Geometry check sheet. Reference: drawing and pictorial views, mm from the part's lowest x, y, z. Coordinates: 2 decimals unless noted, no trailing zeros. Loops run counter-clockwise (first coordinate to the right, second up) from the corner with the lowest first, then second, coordinate; pieces in that order, holes last. Notation, with made-up numbers: M -30,66 L 0,66 A22 ccw 0,102 Z; hole C 45.25,27.25 d3. An arc over 180 degrees is marked long. Write each question's results on one line, items separated by ' | '. Start each with the question number.
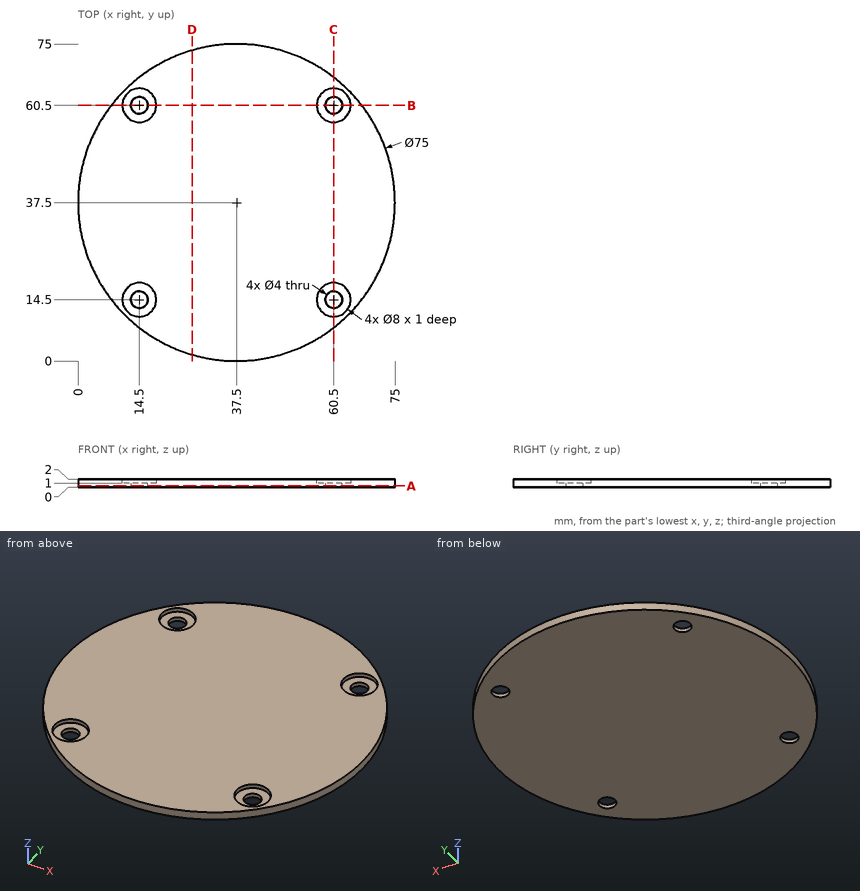
1) Thickness scan on probe 1 along Y at (x, z) = (14.5, 0.7); probe 2 along Y at (x, z) = (57, 1.5). Record the ranges inside material, lowest first.
2) Gauge pin test, flat ends, axial feed: P1, Ø2.5, axis at x = 14.5, y = 60.5, coming from the -Z side; P2, Ø6.5, axis at x = 60.5, y = 60.5, coming from the +Z side. Record the tip position at first contact, or that the pin passes through.
3) Section check B-B (y = 60.5). Enter the section's corners in (x, z).
4) Section check A-A (z = 0.35). Enter the section's corners in (x, y), then the cut area to 3 significant figures.
5) Section check D-D (x = 27). Enter the section's corners in (y, z), then the cut area to 3 significant figures.
Return value:
1) probe 1: y = 7.88 to 12.5, 16.5 to 58.5, 62.5 to 67.12 | probe 2: y = 5.47 to 12.56, 16.44 to 58.56, 62.44 to 69.53
2) P1: passes through | P2: stops at z = 1
3) outline: M 7.88,0 L 12.5,0 L 12.5,1 L 10.5,1 L 10.5,2 L 7.88,2 Z; M 16.5,0 L 58.5,0 L 58.5,1 L 56.5,1 L 56.5,2 L 18.5,2 L 18.5,1 L 16.5,1 Z; M 62.5,0 L 67.12,0 L 67.12,2 L 64.5,2 L 64.5,1 L 62.5,1 Z
4) outline: C 37.5,37.5 d75; hole C 14.5,14.5 d4; hole C 14.5,60.5 d4; hole C 60.5,14.5 d4; hole C 60.5,60.5 d4 | area: 4,370 mm2
5) outline: M 1.5,0 L 73.5,0 L 73.5,2 L 1.5,2 Z | area: 144 mm2
